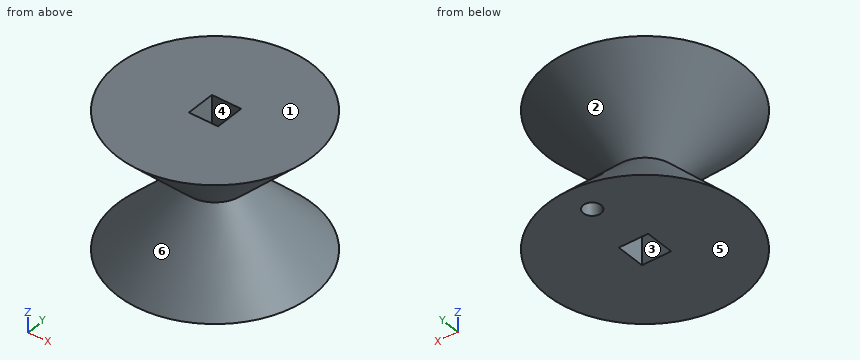
from build123d import *

# Parameters (mm, degrees)
F3_R      = 12.7
F4_R      = 3.81
F2_R      = 12.7
F7_W      = 3.81
F7_H      = 3.81
F8_DEPTH  = 25.4
F9_R      = 1.143
F10_DEPTH = 6.858


with BuildPart() as f5:
    # F3 (on offset) → F5 section 0
    with BuildSketch(Plane.XY.offset(-8.89)):
        Circle(F3_R)
    # F4 (on Top) → F5 section 1
    with BuildSketch(Plane.XY):
        Circle(F4_R)
    loft()

    # F2 (on offset) → F6 section 0
    with BuildSketch(Plane.XY.offset(8.89)):
        Circle(F2_R)
    # F4 (on Top) → F6 section 1
    with BuildSketch(Plane.XY):
        Circle(F4_R)
    loft()

    # F7 (on offset) → F8 (cut)
    with BuildSketch(Plane.XY.offset(8.89)):
        Rectangle(F7_W, F7_H)
    extrude(amount=-F8_DEPTH, mode=Mode.SUBTRACT)

    # F9 (on offset) → F10 (cut)
    with BuildSketch(Plane.XY.offset(-8.89)):
        with Locations((0, 8.72125)):
            Circle(F9_R)
    extrude(amount=F10_DEPTH, mode=Mode.SUBTRACT)


solid = f5.part
The listing builds one solid part. Answer for the finished solid, in the listing's coordinates (mm). Face numbers are marked on the shaded views. A direction names the side the tool comes from. Round coordinates to 2 decimals unless told otherwise and drop trailing zeros. Order: outer loops, then holes, each group sorted by start corner. A loop starts at its lowest first (then second) coordinate and runs counter-clockwise, first axis right, second up. Notation, with made-up numbers: (34.25, -15.75) -> (63.25, -15.75) arc R24 cw to (63.25, 0.25) -> close; hole circle Ø9 at (42, 54.25). An arc over 180 degrees is marked (long way). One line per item, written item: value.
Item 1: For the marked faces 4, 5 and 6, determine the directions among +Z, -Z, +X, -X, +Y, -Y from which every point of the face is accessible in a straight line to the end or side of a thin tool.
Taken from the geometry:
face 4: +Z, -Z
face 5: -Z, +X, -X, +Y, -Y
face 6: none
Item 2: Find section C-C, the plane z = 6.25. Give the vertices of the cut face in (x, y) (3 decimals).
Taken from the geometry:
outline: circle Ø20.12 at (0, 0); hole (-1.905, -1.905) -> (1.905, -1.905) -> (1.905, 1.905) -> (-1.905, 1.905) -> close
Item 3: For a pull along Z with two mould halves and no side action, classify the marked faces 1, 2 and 3 as released by +Z, released by -Z, zero draft, split by the parting line, or undercut.
Taken from the geometry:
face 1: released by +Z
face 2: undercut
face 3: zero draft
Item 4: Given P1, Ø1, axis at y = -5, z = 3, coming from the +X side; P2, Ø3, axis at x = -7, z = -5.5, coming from the -Y side; P3, Ø3, axis at x = 0.5, z = 3, coming from the +Y side, each flat-ended and moving along its own axis, determine where each tip first touches the part or whether it passes through.
Taken from the geometry:
P1: stops at x = 5.47
P2: stops at y = -8.57
P3: stops at y = 8.3
Item 5: Straight lines are drawn through the part: L1, parallel to Y at x = 0, z = -7 (3 decimals); L2, parallel to X at y = 1, z = -4 (3 decimals); L3, parallel to Z at x = -7, y = 2.25. For each, find the intervals that lie inside material, in ascending order.
Taken from the geometry:
L1: y = -10.81 to -1.905, 1.905 to 7.578, 9.864 to 10.81
L2: x = -7.746 to -1.905, 1.905 to 7.746
L3: z = -8.89 to -3.54, 3.54 to 8.89
Item 6: Find section B-B, the plane x = 0. Give the vertices of the cut face in (y, z) (3 decimals).
Taken from the geometry:
outline: (-12.7, -8.89) -> (-1.905, -8.89) -> (-1.905, 8.89) -> (-12.7, 8.89) -> (-3.81, 0) -> close; (1.905, -8.89) -> (7.578, -8.89) -> (7.578, -3.768) -> (3.81, 0) -> (12.7, 8.89) -> (1.905, 8.89) -> close; (9.864, -8.89) -> (12.7, -8.89) -> (9.864, -6.054) -> close
Item 7: Find section A-A, the plane z = 3.5. Give the vertices of the cut face in (x, y) (3 decimals), then the cut area to 3 significant figures.
Taken from the geometry:
outline: circle Ø14.62 at (0, 0); hole (-1.905, -1.905) -> (1.905, -1.905) -> (1.905, 1.905) -> (-1.905, 1.905) -> close
area: 153 mm2
